Check sheet for the modelled part. Datum: model origin and axes. Units: mm. Face numbers are marked on the shaded views. A direction names the side the tool comes from. Round coordinates to 2 decimals unless told otherwise and drop trailing zeros. Loops run counter-clockwise (first coordinate to the right, second up) from the corner with the lowest first, then second, coordinate; pieces in that order, holes last. Notation, with made-up numbers: (-6.5, -16) -> (52.5, -16) arc R20 cw to (52.5, 0) -> close; hole circle Ø1 at (-16.75, 26.25). An arc over 180 degrees is marked (long way). Return JSON: item names as keys, results as strings.
from build123d import *

# Parameters (mm, degrees)
F0_R     = 38.1
F1_DEPTH = 12.7
F2_R     = 38.1
F2_R_2   = 31.75
F3_DEPTH = 6.35
F4_R     = 3.175
F5_DEPTH = 12.701
F7_DEPTH = 12.701


with BuildPart() as f1:
    # F0 (on Top) → F1 (new body)
    with BuildSketch(Plane.XY):
        Circle(F0_R)
    extrude(amount=F1_DEPTH)

    # F2 (on face) → F3 (cut)
    with BuildSketch(Plane(origin=(0, 0, 0), x_dir=(1, 0, 0), z_dir=(0, 0, -1))):
        Circle(F2_R)
        Circle(F2_R_2, mode=Mode.SUBTRACT)
    extrude(amount=-F3_DEPTH, mode=Mode.SUBTRACT)

    # F4 (on face) → F5 (cut, through all)
    with BuildSketch(Plane.XY.offset(12.7)):
        Circle(F4_R)
    extrude(amount=-F5_DEPTH, mode=Mode.SUBTRACT)

    # F6 (on face) → F7 (cut, through all)
    with BuildSketch(Plane.XY.offset(12.7)):
        with BuildLine():
            Line((-3.2004, 31.75), (-3.2004, 12.7))
            ThreePointArc((-3.2004, 12.7), (0, 9.4996), (3.2004, 12.7))
            Line((3.2004, 12.7), (3.2004, 31.75))
            ThreePointArc((3.2004, 31.75), (0, 34.9504), (-3.2004, 31.75))
        make_face()
    extrude(amount=-F7_DEPTH, mode=Mode.SUBTRACT)


solid = f1.part
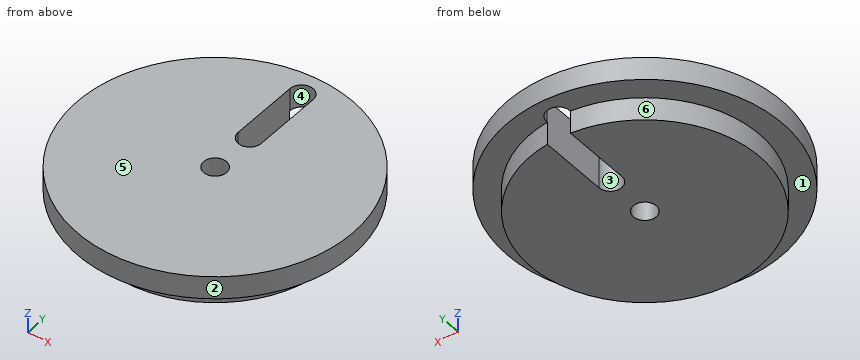
Q1. Tool access check on the marked faces 4, 5 and 6. Record the directions out of +Z, -Z, +X, -X, +Y, -Y that give a thin tool (end or side, any length) a straight path to the whole face; none if there is none.
Results list:
{"face 4": "+Z, -Z", "face 5": "+Z, +X, -X, +Y, -Y", "face 6": "-Z"}
Q2. Section check C-C (z = 1.25). Record the boundary of the cut face in (x, y) (3 decimals), then the cut area to 3 significant figures.
Results list:
{"outline": "(-3.2, 12.7) -> (-3.2, 31.588) arc R31.75 ccw (long way) to (3.2, 31.588) -> (3.2, 12.7) arc R3.2 cw to start; hole circle Ø6.35 at (0, 0)", "area": "3,000 mm^2"}
Q3. Section check A-A (y = 0). Record the boundary of the cut face in (x, z) (3 decimals), then the cut area to 3 significant figures.
Results list:
{"outline": "(-38.1, 6.35) -> (-31.75, 6.35) -> (-31.75, 0) -> (-3.175, 0) -> (-3.175, 12.7) -> (-38.1, 12.7) -> close; (3.175, 0) -> (31.75, 0) -> (31.75, 6.35) -> (38.1, 6.35) -> (38.1, 12.7) -> (3.175, 12.7) -> close", "area": "806 mm^2"}
Q4. Material ranges on line 1 (Y direction, x = 0, z = 10.25) (3 decimals); line 2 (X direction, y = 31.5, z = 9.5); line 3 (Z direction, x = 21.5, y = 24), recorded low to high.
Results list:
{"line 1": "-38.1 to -3.175, 3.175 to 9.5, 34.95 to 38.1", "line 2": "-21.43 to -3.2, 3.2 to 21.43", "line 3": "6.35 to 12.7"}
Q5. Section check B-B (x = 0). Record the boundary of the cut face in (y, z) (3 decimals).
Results list:
{"outline": "(-38.1, 6.35) -> (-31.75, 6.35) -> (-31.75, 0) -> (-3.175, 0) -> (-3.175, 12.7) -> (-38.1, 12.7) -> close; (3.175, 0) -> (9.5, 0) -> (9.5, 12.7) -> (3.175, 12.7) -> close; (34.95, 6.35) -> (38.1, 6.35) -> (38.1, 12.7) -> (34.95, 12.7) -> close"}
Q6. Go/stop test with flat-tipped pins: pin 1 (6.5 mm diameter, centred on y = 23.5, z = 7.5, fed in from +X); pin 2 (3 mm diameter, centred on x = 6, y = 24, fed in from -Z); pin 3 (4 mm diameter, centred on y = -20.5, z = 4, fed in from +X); pin 4 (1.5 mm diameter, centred on x = -5.5, z = 6.5, fed in from -Y). Record where each tip stops, or that it passes through.
Results list:
{"pin 1": "x = 32.27", "pin 2": "z = 0", "pin 3": "x = 25.8", "pin 4": "y = -37.8"}
Q7. Draft check along Y on the marked faces 1, 2 and 3. Enter one of: released by +Y, released by -Y, zero draft, split by the parting line, or undercut.
Results list:
{"face 1": "zero draft", "face 2": "split by the parting line", "face 3": "undercut"}
Q8. Section check D-D (z = 10.5). Record the boundary of the cut face in (x, y) (3 decimals).
Results list:
{"outline": "circle Ø76.2 at (0, 0); hole (-3.2, 12.7) arc R3.2 ccw to (3.2, 12.7) -> (3.2, 31.75) arc R3.2 ccw to (-3.2, 31.75) -> close; hole circle Ø6.35 at (0, 0)"}
